Geometry check sheet. Reference: the model listing, model coordinates, mm. A direction names the side the tool comes from. Coordinates: 2 decimals unless noted, no trailing zeros. Order: outer loops, then holes, each group sorted by start corner. A loop starts at its lowest first (then second) coordinate and runs counter-clockwise, first axis right, second up. Notation, with made-up numbers: M -19.5,25.25 L -11.5,25.25 A17 cw -11.5,46.25 Z; hole C 11.25,-27 d3. An arc over 180 degrees is marked long. Use CSV: the item, a comma, the result in double quotes. Start each with the question number.
Autodesk Fusion 360 part; units mm, degrees
sketch "Sketch1" plane through (0, 0, 0) normal (0, 0, 1) x (1, 0, 0)
  line L0 (0, 0) -> (11.8, 0) construction
  line L1 (2, 0) -> (2, 4.9481) construction
  line L2 (9.6021, 2.8908) -> (3.4309, 4.603)
  arc A0 (0.3331, 2.7838) -> (0, 0) centre (11.8, 0) ccw
  arc A1 (11.8, 0) -> (9.6021, 2.8908) centre (8.8, 0) ccw
  arc A2 (3.4309, 4.603) -> (0.3331, 2.7838) centre (2.7625, 2.194) ccw
  arc A3 (0, 0) -> (0.3331, -2.7838) centre (11.8, 0) ccw
  arc A4 (0.3331, -2.7838) -> (3.4309, -4.603) centre (2.7625, -2.194) ccw
  line L3 (9.6021, -2.8908) -> (3.4309, -4.603)
  arc A5 (9.6021, -2.8908) -> (11.8, 0) centre (8.8, 0) ccw
  circle A6 centre (6, 0) radius 1
  circle A7 centre (2.5, 0) radius 1
  circle A8 centre (9.5, 0) radius 1
  arc A9 (-2, 0) -> (-1.6105, -3.2556) centre (11.8, 0) ccw
  arc A10 (-1.6105, -3.2556) -> (3.9656, -6.5302) centre (2.7625, -2.194) ccw
  line L4 (10.1368, -4.818) -> (3.9656, -6.5302)
  arc A11 (10.1368, -4.818) -> (13.8, 0) centre (8.8, 0) ccw
  arc A12 (13.8, 0) -> (10.1368, 4.818) centre (8.8, 0) ccw
  line L5 (10.1368, 4.818) -> (3.9656, 6.5302)
  arc A13 (3.9656, 6.5302) -> (-1.6105, 3.2556) centre (2.7625, 2.194) ccw
  arc A14 (-1.6105, 3.2556) -> (-2, 0) centre (11.8, 0) ccw
  dimension "d1" = 11.8
  dimension "d2" = 6
  dimension "d4" = 5
  dimension "d5" = 2
  dimension "d6" = 6
  dimension "d7" = 2
  dimension "d8" = 2.5
  dimension "d9" = 2
  dimension "d10" = 3.5
  dimension "d11" = 2
extrude "Extrude1" add sketch "Sketch1" along normal blind 2.6 contours L2 A0 A1 A2 A3 A4 L3 A5
extrude "Extrude2" add sketch "Sketch1" along normal blind 0.6 contours A9 A10 L4 A11 A12 L5 A13 A14
fillet "Fillet1" radius 0.2 6 edges at (6.5165, 3.7469, 2.6) (1.4965, 4.3498, 2.6) (0, 0, 2.6) (1.4965, -4.3498, 2.6) (6.5165, -3.7469, 2.6) (11.8, 0, 2.6)
1) Gauge pin test, flat ends, axial feed: P1, Ø1.6, axis at x = 6, y = 0, coming from the +Z side; P2, Ø1, axis at x = 6, y = -4.5, coming from the -Z side; P3, Ø1, axis at y = -3.5, z = 1, coming from the +X side. Record the tip position at first contact, or that the pin passes through.
2) Set-up check for faces 4 (the face through (6.45, -3.94, 0.6)), 5 (the face through (6.56, -3.735, 1.487)), 6 (the face through (6.56, 3.735, 1.487)): record each of +Z, -Z, +X, -X, +Y, -Y from which the full face is reachable in a straight line by a thin tool's end or side.
3) Section check A-A on z = 0.95. Record the boundary of the cut face in (x, y).
4) Draft check along X on faces 1 (the face through (4.6, 0.1, 2.6)), 2 (the face through (1.5, 0, 1.3)), 3 (the face through (1.521, -4.364, 1.487)). Enter one of: +X half, -X half, draft (parallel to the pull), parting line (faces both ways), or undercut.
5) Material ranges on line 1 along X through (y, z) = (0.25, 0.65); line 2 along Z through (x, y) = (-0.75, 0); line 3 along Y through (x, z) = (9.5, 1.4), recorded low to high.
Results are:
1,P1,"passes through"
1,P2,"stops at z = 0"
1,P3,"stops at x = 12.64"
2,face 4,"+Z"
2,face 5,"+Z, +X, -Y"
2,face 6,"+Z, +X, +Y"
3,outline,"M 0,0 A11.8 ccw 0.33,-2.78 A2.5 ccw 3.43,-4.6 L 9.6,-2.89 A3 ccw 11.8,0 A3 ccw 9.6,2.89 L 3.43,4.6 A2.5 ccw 0.33,2.78 A11.8 ccw Z; hole C 2.5,0 d2; hole C 6,0 d2; hole C 9.5,0 d2"
4,face 1,"draft"
4,face 2,"undercut"
4,face 3,"parting line"
5,line 1,"x = 0 to 1.53, 3.47 to 5.03, 6.97 to 8.53, 10.47 to 11.79"
5,line 2,"z = 0 to 0.6"
5,line 3,"y = -2.92 to -1, 1 to 2.92"
